Here's how the part is built. I have some questions about the finished solid (model axes, mm). Face numbers are marked on the shaded views. Round coordinates to 2 decimals unless told otherwise and drop trailing zeros. Write each loop counter-clockwise with the first axis right and the second up, starting at its lowest first coordinate (ties: lowest second). Pieces come first, ordered by that corner, then holes. Notation, with made-up numbers: (0, 4.5) - (49, 4.5) arc R5 ccw to (49, 10.5) - close; hole circle Ø10 at (1, -33.5). An arc over 180 degrees is marked (long way). One line per question, with ' | ' between items. Start each with the question number.
(1) Imagine slicing it at D-D (x = -7). Write out the boundary of the cut face in (y, z).
(2) Imagine slicing it at A-A (x = 0). Write out the boundary of the cut face in (y, z).
(3) Imagine slicing it at C-C (z = 0.8). Write out the boundary of the cut face in (x, y).
(4) Will these pins go through, and if not, where does the flat tip stop? pin 1 (1.5 mm diameter, centred on y = -2.5, z = 2, fed in from -X); pin 2 (2.5 mm diameter, centred on x = -22, y = 0, fed in from +Z); pin 3 (1.5 mm diameter, centred on y = 19, z = 1, fed in from +X).
(5) If I drill on L1, parallel to Y at x = 0, z = 3.15; L2, parallel to Y at x = 22, z = 2.9; L3, parallel to X at y = -1.5, z = 4, over which ranges is the centre line in solid material (lowest first)?
(6) Imagine slicing it at B-B (y = 0). Write out the boundary of the cut face in (x, z).
(7) Thinking about a two-plate mould opening in X: for the marked faces 1, 2 and 3, which applies, pulls with the +X half, pulls with the -X half, needs draft (parallel to the pull), parting line crosses it, or undercut?
from build123d import *

# Parameters (mm, degrees)
SKETCH1_R           = 25
SKETCH1_R_2         = 7.5
BOSS_EXTRUDE1_DEPTH = 5
SKETCH2_R           = 2
CUT_EXTRUDE1_DEPTH  = 5


with BuildPart() as part:
    # Sketch1 → Boss-Extrude1 (new body)
    with BuildSketch(Plane.XY):
        Circle(SKETCH1_R)
        Circle(SKETCH1_R_2, mode=Mode.SUBTRACT)
    extrude(amount=BOSS_EXTRUDE1_DEPTH)

    # Sketch2 → Cut-Extrude1 (cut)
    with BuildSketch(Plane.XY.offset(5)):
        with Locations((0, 22)):
            Circle(SKETCH2_R)
        with Locations((22, 0)):
            Circle(SKETCH2_R)
        with Locations((-22, 0)):
            Circle(SKETCH2_R)
        with BuildLine():
            Line((-22.24968915, -11.39961985), (22.24968915, -11.39961985))
            ThreePointArc((22.24968915, -11.39961985), (0, -25), (-22.24968915, -11.39961985))
        make_face()
    extrude(amount=-CUT_EXTRUDE1_DEPTH, mode=Mode.SUBTRACT)


solid = part.part
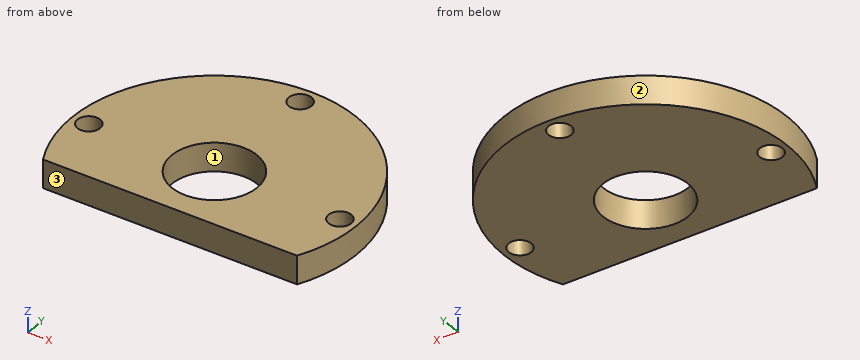
Check sheet entries:
1) outline: (-11.4, 0) - (-2.69, 0) - (-2.69, 5) - (-11.4, 5) - close; (2.69, 0) - (24, 0) - (24, 5) - (2.69, 5) - close
2) outline: (-11.4, 0) - (-7.5, 0) - (-7.5, 5) - (-11.4, 5) - close; (7.5, 0) - (20, 0) - (20, 5) - (7.5, 5) - close; (24, 0) - (25, 0) - (25, 5) - (24, 5) - close
3) outline: (-22.25, -11.4) - (22.25, -11.4) arc R25 ccw (long way) to start; hole circle Ø4 at (-22, 0); hole circle Ø15 at (0, 0); hole circle Ø4 at (0, 22); hole circle Ø4 at (22, 0)
4) pin 1: x = -24.94 | pin 2: through | pin 3: x = 17.09
5) L1: -11.4 to -7.5, 7.5 to 20, 24 to 25 | L2: -11.4 to -2, 2 to 11.87 | L3: -24.95 to -23.32, -20.68 to -7.35, 7.35 to 20.68, 23.32 to 24.95
6) outline: (-25, 0) - (-24, 0) - (-24, 5) - (-25, 5) - close; (-20, 0) - (-7.5, 0) - (-7.5, 5) - (-20, 5) - close; (7.5, 0) - (20, 0) - (20, 5) - (7.5, 5) - close; (24, 0) - (25, 0) - (25, 5) - (24, 5) - close
7) face 1: undercut | face 2: parting line crosses it | face 3: needs draft
